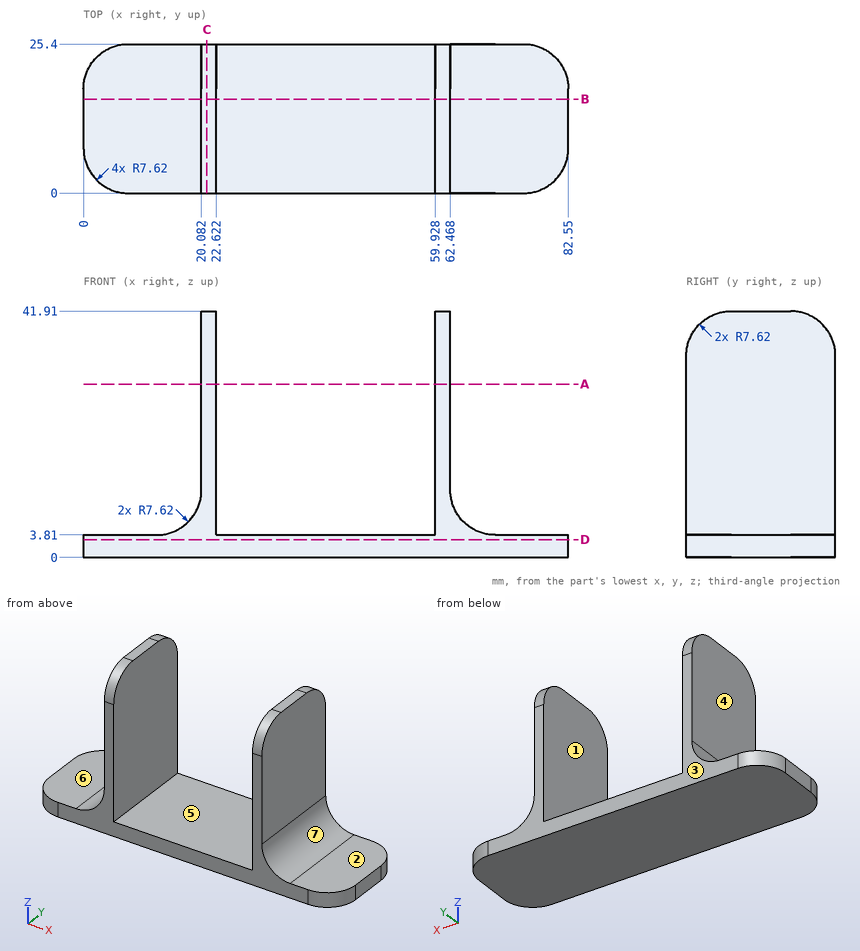
Geometry: see drawing. Coordinates: mm, zero at the bounding-box minimum. A direction names the side the tool comes from. Give positions to 0.01 mm unless a question says otherwise; leave off trailing zeros. Order: outer loops, then holes, each group sorted by start corner. A loop starts at its lowest first (then second) coordinate and runs counter-clockwise, first axis right, second up. Notation, with made-up numbers: (-33.75, 69.25) - (-0.75, 69.25) arc R35 cw to (-0.75, 107.25) - close; hole circle Ø2 at (21.5, 63). An arc over 180 degrees is marked (long way). Write each question's results on one line, items separated by ' | '.
Item 1: Section A-A (z = 29.5). Return loops of the section in (x, y).
A:
outline: (20.08, 0) - (22.62, 0) - (22.62, 25.4) - (20.08, 25.4) - close; (59.93, 0) - (62.47, 0) - (62.47, 25.4) - (59.93, 25.4) - close
Item 2: Draft query along X for the marked faces 4, 5, 6 and 7. Return one class per face: released by +X, released by -X, zero draft, split by the parting line, or undercut.
A:
face 4: released by -X | face 5: undercut | face 6: zero draft | face 7: released by +X
Item 3: Material intervals for line 1 along X through (y, z) = (9.5, 29.5); line 2 along Z through (x, y) = (73.5, 3); line 3 along X through (y, z) = (2, 9.5), sorted ascending.
A:
line 1: x = 20.08 to 22.62, 59.93 to 62.47 | line 2: z = 0 to 3.81 | line 3: x = 19.83 to 22.62, 59.93 to 62.72
Item 4: Section C-C (x = 21). Return loops of the section in (y, z).
A:
outline: (0, 0) - (25.4, 0) - (25.4, 34.29) arc R7.62 ccw to (17.78, 41.91) - (7.62, 41.91) arc R7.62 ccw to (0, 34.29) - close
Item 5: Section B-B (y = 16). Return loops of the section in (x, z), and give its area (3 significant figures).
A:
outline: (0, 0) - (82.55, 0) - (82.55, 3.81) - (70.09, 3.81) arc R7.62 cw to (62.47, 11.43) - (62.47, 41.91) - (59.93, 41.91) - (59.93, 3.81) - (22.62, 3.81) - (22.62, 41.91) - (20.08, 41.91) - (20.08, 11.43) arc R7.62 cw to (12.46, 3.81) - (0, 3.81) - close | area: 533 mm^2
Item 6: Section D-D (z = 3). Return loops of the section in (x, y), and give its area (3 significant figures).
A:
outline: (0, 7.62) arc R7.62 ccw to (7.62, 0) - (74.93, 0) arc R7.62 ccw to (82.55, 7.62) - (82.55, 17.78) arc R7.62 ccw to (74.93, 25.4) - (7.62, 25.4) arc R7.62 ccw to (0, 17.78) - close | area: 2,050 mm^2
Item 7: Contact query for flat-ended pins moving along their axis: pin 1 Ø10 at (y, z) = (14.5, 11) entering from -X; pin 2 Ø3 at (y, z) = (4.5, 26.5) entering from -X; pin 3 Ø3 at (x, y) = (30.5, 17) entering from +Z; pin 4 Ø8 at (x, z) = (38, 11.5) entering from -Y. Output: stop coordinate, or through.
A:
pin 1: stops at x = 17.81 | pin 2: stops at x = 20.08 | pin 3: stops at z = 3.81 | pin 4: passes through
Item 8: Access query for the marked faces 1, 2 and 3. Directions: +Z, -Z, +X, -X, +Y, -Y. A direction counts if a zero-diameter tool reaches every point of the face in a straight line with its end or side. Return the directions, or none.
A:
face 1: +Z, +Y, -Y | face 2: +Z, +X, +Y, -Y | face 3: +Z, -Z, +X, -X, +Y
